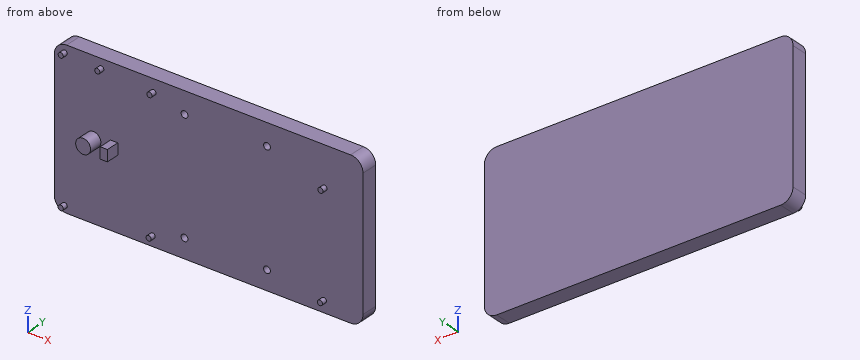
from build123d import *

# Parameters (mm, degrees)
EXTRUDE_1_DEPTH     = 8
SKETCH_2_6_R        = 1.25
EXTRUDE_6_DEPTH     = 2.5
SKETCH_2_7_R        = 1.65
CUT_EXTRUDE_1_DEPTH = 4
SKETCH_2_R          = 3.6
SKETCH_2_W          = 3.5
SKETCH_2_H          = 5.5
EXTRUDE_7_DEPTH     = 6.5


with BuildPart() as part:
    # Sketch 1 → Extrude 1 (new body)
    with BuildSketch(Plane(origin=(0, 0, 0), x_dir=(1, 0, 0), z_dir=(0, 1, 0))):
        with BuildLine():
            Line((6, 0), (143.8, 0))
            ThreePointArc((143.8, 0), (148.042640687, -1.757359313), (149.8, -6))
            Line((149.8, -6), (149.8, -68.8))
            ThreePointArc((149.8, -68.8), (148.042640687, -73.042640687), (143.8, -74.8))
            Line((143.8, -74.8), (6, -74.8))
            ThreePointArc((6, -74.8), (1.757359313, -73.042640687), (0, -68.8))
            Line((0, -68.8), (0, -6))
            ThreePointArc((0, -6), (1.757359313, -1.757359313), (6, 0))
        make_face()
    extrude(amount=EXTRUDE_1_DEPTH)

    # Sketch 2_6 → Extrude 6 (add)
    with BuildSketch(Plane(origin=(0, 0, 0), x_dir=(-1, 0, 0), z_dir=(0, -1, 0))):
        with Locations(Location((-130.8, -5.6, 0), (0, 0, 90))):
            Circle(SKETCH_2_6_R)
        with Locations(Location((-131.1, -55.65, 0), (0, 0, 90))):
            Circle(SKETCH_2_6_R)
        with Locations(Location((-47.7, -4.85, 0), (0, 0, 90))):
            Circle(SKETCH_2_6_R)
        with Locations(Location((-48.1, -68.75, 0), (0, 0, 90))):
            Circle(SKETCH_2_6_R)
        with Locations(Location((-22.8, -70.3, 0), (0, 0, 90))):
            Circle(SKETCH_2_6_R)
        with Locations(Location((-5.05, -71.05, 0), (0, 0, 90))):
            Circle(SKETCH_2_6_R)
        with Locations(Location((-5.05, -3.25, 0), (0, 0, 90))):
            Circle(SKETCH_2_6_R)
    extrude(amount=EXTRUDE_6_DEPTH)

    # Sketch 2_7 → Cut-Extrude 1 (cut)
    with BuildSketch(Plane(origin=(0, 0, 0), x_dir=(-1, 0, 0), z_dir=(0, -1, 0))):
        with Locations(Location((-103.2, -9.35, 0), (0, 0, 90))):
            Circle(SKETCH_2_7_R)
        with Locations(Location((-103.2, -64.25, 0), (0, 0, 90))):
            Circle(SKETCH_2_7_R)
        with Locations(Location((-63.2, -64.25, 0), (0, 0, 90))):
            Circle(SKETCH_2_7_R)
        with Locations(Location((-63.2, -9.35, 0), (0, 0, 90))):
            Circle(SKETCH_2_7_R)
    extrude(amount=-CUT_EXTRUDE_1_DEPTH, mode=Mode.SUBTRACT)

    # Sketch 2 → Extrude 7 (add)
    with BuildSketch(Plane(origin=(0, 0, 0), x_dir=(-1, 0, 0), z_dir=(0, -1, 0))):
        with Locations(Location((-19, -37.4, 0), (0, 0, 270))):
            Circle(SKETCH_2_R)
        with Locations((-29.05, -37.4)):
            Rectangle(SKETCH_2_W, SKETCH_2_H)
    extrude(amount=EXTRUDE_7_DEPTH)


solid = part.part
Model file for the job. Use its own axes, mm. Coordinates: 2 decimals unless noted, no trailing zeros. Loops run counter-clockwise (first coordinate to the right, second up) from the corner with the lowest first, then second, coordinate; pieces in that order, holes last. Notation, with made-up numbers: (38, 16) -> (54, 16) arc R25 ccw to (54, 55) -> close; hole circle Ø5 at (35.25, 10). An arc over 180 degrees is marked (long way). Use one line per item in the form item = value. Start each with the question number.
(1) Cut at D-D on x = 67. Give the cut face in (y, z), and give its area (3 significant figures).
(2) Cut at A-A on x = 19. Give the cut face in (y, z).
(3) Cut at B-B on z = 37.4. Give the cut face in (x, y), and give its area (3 significant figures).
(4) Flat gauge pins, fed straight in: pin 1 (1 mm diameter, centred on x = 104, z = 65, fed in from -Y); pin 2 (1.2 mm diameter, centred on x = 4.5, z = 71.5, fed in from -Y); pin 3 (6 mm diameter, centred on x = 90, z = 22, fed in from -Y). Where does each tip first touch, or does it go through?
(5) Cut at C-C on z = 13.5. Give the cut face in (x, y), and give its area (3 significant figures).
(6) Probe probe 1 along Z at (x, y) = (103.2, 1.35); probe 2 along X at (y, z) = (3.1, 64.25); probe 3 along Y at (x, z) = (110.5, 55). List the from-to ranges inside material, lowest first. Write a range as from..to.
Values:
q1.outline = (0, 0) -> (8, 0) -> (8, 74.8) -> (0, 74.8) -> close
q1.area = 598 mm2
q2.outline = (-6.5, 33.8) -> (0, 33.8) -> (0, 0) -> (8, 0) -> (8, 74.8) -> (0, 74.8) -> (0, 41) -> (-6.5, 41) -> close
q3.outline = (0, 0) -> (15.4, 0) -> (15.4, -6.5) -> (22.6, -6.5) -> (22.6, 0) -> (27.3, 0) -> (27.3, -6.5) -> (30.8, -6.5) -> (30.8, 0) -> (149.8, 0) -> (149.8, 8) -> (0, 8) -> close
q3.area = 1,270 mm2
q4.pin_1 = 4
q4.pin_2 = -2.5
q4.pin_3 = 0
q5.outline = (0, 0) -> (149.8, 0) -> (149.8, 8) -> (0, 8) -> close
q5.area = 1,200 mm2
q6.probe_1 = 0..7.7, 11..62.6, 65.9..74.8
q6.probe_2 = 0..61.55, 64.85..101.55, 104.85..149.8
q6.probe_3 = 0..8
